Can you work these out from the model? Positions are in its coordinate system, mm. Face numbers are marked on the shaded views. Give positions to 0.01 mm unless a question says otherwise; leave off trailing zeros. Loops run counter-clockwise (first coordinate to the right, second up) from the corner with the lowest first, then second, coordinate; pieces in that order, holes last. Notation, with made-up numbers: (75.25, 4.5) -> (98.25, 4.5) arc R25 cw to (98.25, 27.5) -> close; hole circle Ø10 at (-11.75, -37). An arc over 180 degrees is marked (long way). Return JSON: item names as keys, results as strings. Group by question number.
Q1. Thinking about a two-plate mould opening in Y: for the marked faces 1, 2, 3 and 4, which applies, pulls with the +Y half, pulls with the -Y half, needs draft (parallel to the pull), parting line crosses it, or undercut?
Q2. Will these pins go through, and if not, where does the flat tip stop? pin 1 (1.5 mm diameter, centred on y = 361.5, z = 285.5, fed in from +X); pin 2 (21 mm diameter, centred on x = -36.23, z = 317.5, fed in from +Y); pin 3 (1.5 mm diameter, centred on x = -363, y = -261, fed in from +Z).
Q3. Suppose I cut it at A-A, the plane x = 341. Please give me the cut outline in (y, z), and give its area (3 significant figures).
Q4. Suppose I cut it at D-D, the plane x = -844.5. Please give me the cut outline in (y, z).
Q5. Suppose I cut it at B-B, the plane y = 195.5. Please give me the cut outline in (x, z), and give its area (3 significant figures).
Q6. Suppose I cut it at C-C, the plane y = 294.5. Please give me the cut outline in (x, z).
Q7. I need wall thicknesses on line 1 along X through (y, z) = (-340, 317); line 2 along Y through (x, z) = (427, 277); line 3 along Z through (x, y) = (798.5, 22). Which ranges of each line are inside material? Lowest first, please. Write a range as [from, to].
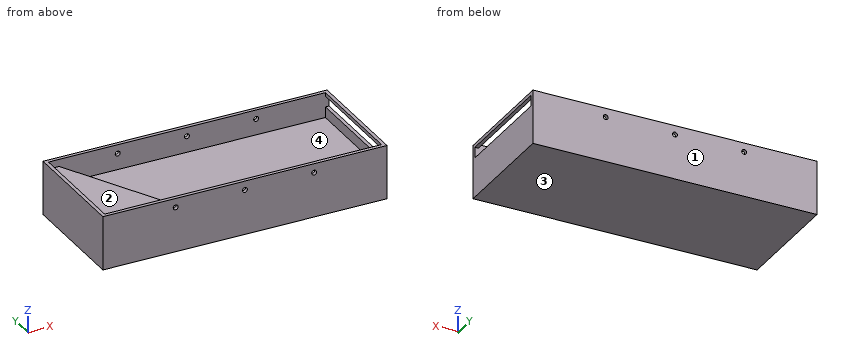
Solid Edge part; units mm, degrees
sketch "Sketch1" plane through (0, 0, 0) normal (0, 0, 1) x (1, 0, 0)
  line L0 (-1039.5328, -355.3891) -> (967.0672, -355.3891)
  line L1 (967.0672, -355.3891) -> (967.0672, 457.4109)
  line L2 (967.0672, 457.4109) -> (-1039.5328, 457.4109)
  line L3 (-1039.5328, 457.4109) -> (-1039.5328, -355.3891)
extrude "Protrusion1" add sketch "Sketch1" along normal blind 381
sketch "Sketch2" plane through (-61.6328, 25.6109, 381) normal (0, 0, 1) x (1, 0, 0)
  line L0 (-469.9, -355.6) -> (-876.3, 406.4)
  line L1 (1003.3, 406.4) -> (-876.3, 406.4)
  line L2 (1003.3, -355.6) -> (1003.3, 406.4)
  line L3 (-469.9, -355.6) -> (1003.3, -355.6)
extrude "ExtrudedCutout_1" cut sketch "Sketch2" along normal mid plane 355.6
sketch "Sketch3" plane through (-36.2328, 51.0109, 381) normal (0, 0, 1) x (1, 0, 0)
  line L0 (-495.3, -381) -> (-901.7, 381)
  line L1 (-901.7, 381) -> (-977.9, 381)
  line L2 (-977.9, 381) -> (-977.9, -381)
  line L3 (-977.9, -381) -> (-495.3, -381)
extrude "ExtrudedCutout_2" cut sketch "Sketch3" along normal mid plane 101.6
sketch "Sketch4" plane through (941.6672, 51.0109, 292.1) normal (-1, 0, 0) x (0, -1, 0)
  line L0 (-381, 63.5) -> (381, 63.5)
  line L1 (381, 63.5) -> (381, -12.7)
  line L2 (381, -12.7) -> (-381, -12.7)
  line L3 (-381, -12.7) -> (-381, 63.5)
extrude "ExtrudedCutout_3" cut sketch "Sketch4" along normal mid plane 909.4412
sketch "Sketch5" plane through (-23.5328, 432.0109, 292.1) normal (0, -1, 0) x (1, 0, 0)
  circle A0 centre (-501.65, 25.4) radius 17.4625
  circle A1 centre (-12.7, 25.4) radius 17.4625
  circle A2 centre (476.25, 25.4) radius 17.4625
extrude "ExtrudedCutout_5" cut sketch "Sketch5" along normal blind 2228.9962 and the other way blind 429.4298
properties material "Wood, balsa"
Ans:
{
 "1": {"face 1": "pulls with the +Y half", "face 2": "undercut", "face 3": "needs draft", "face 4": "undercut"},
 "2": {"pin 1": "stops at x = -899.93", "pin 2": "passes through", "pin 3": "stops at z = 203.2"},
 "3": {"outline": "(-355.39, 0) -> (457.41, 0) -> (457.41, 381) -> (432.01, 381) -> (432.01, 203.2) -> (-329.99, 203.2) -> (-329.99, 381) -> (-355.39, 381) -> close", "area": "174,000 mm^2"},
 "4": {"outline": "(-355.39, 0) -> (457.41, 0) -> (457.41, 381) -> (432.01, 381) -> (432.01, 203.2) -> (256.82, 203.2) -> (256.82, 330.2) -> (-329.99, 330.2) -> (-329.99, 381) -> (-355.39, 381) -> close"},
 "5": {"outline": "(-1039.53, 0) -> (967.07, 0) -> (967.07, 279.4) -> (941.67, 279.4) -> (941.67, 203.2) -> (-811.79, 203.2) -> (-811.79, 330.2) -> (-1014.13, 330.2) -> (-1014.13, 381) -> (-1039.53, 381) -> close; (941.67, 355.6) -> (967.07, 355.6) -> (967.07, 381) -> (941.67, 381) -> close", "area": "441,000 mm^2"},
 "6": {"outline": "(-1039.53, 0) -> (967.07, 0) -> (967.07, 279.4) -> (941.67, 279.4) -> (941.67, 203.2) -> (-864.59, 203.2) -> (-864.59, 330.2) -> (-1014.13, 330.2) -> (-1014.13, 381) -> (-1039.53, 381) -> close; (941.67, 355.6) -> (967.07, 355.6) -> (967.07, 381) -> (941.67, 381) -> close"},
 "7": {"line 1": "x = [-1039.53, -542.64], [-507.73, -53.69], [-18.78, 435.26], [470.17, 967.07]", "line 2": "y = [-355.39, -329.99], [432.01, 457.41]", "line 3": "z = [0, 203.2]"}
}
